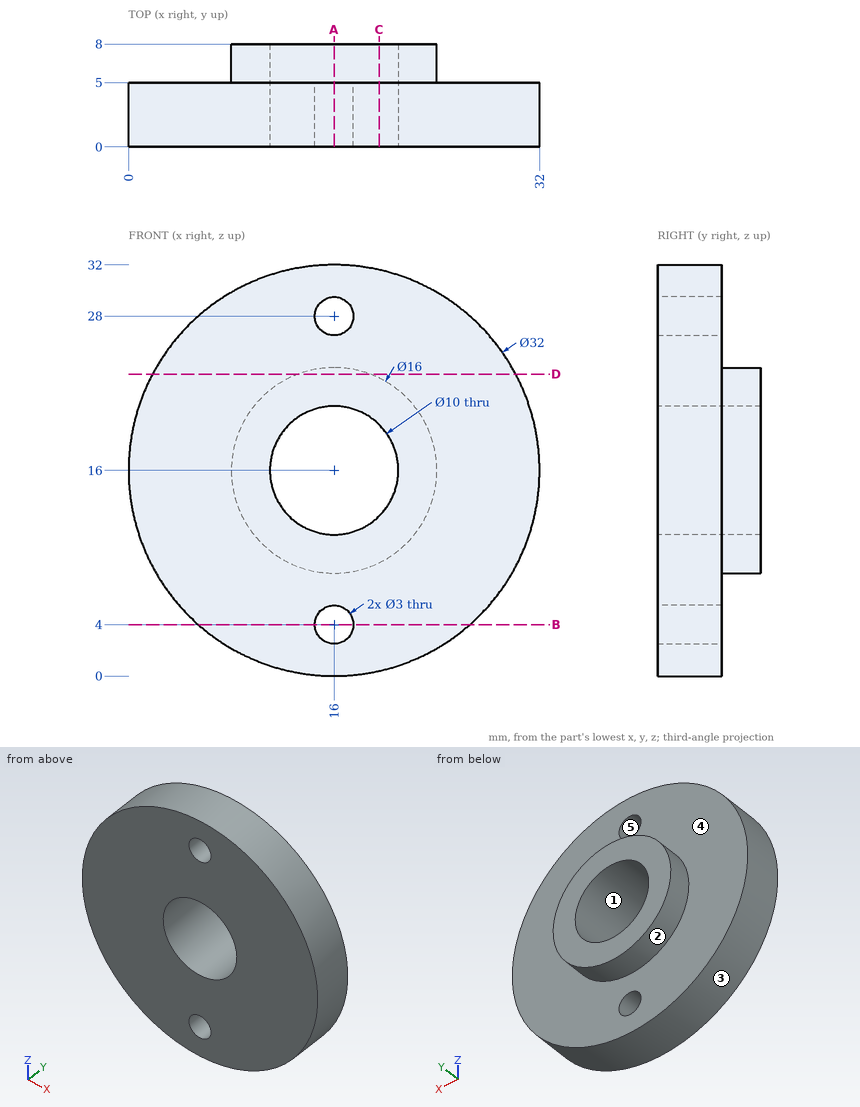
Can you work these out from the drawing? Everything is in mm from the part's minimum corner. A direction names the side the tool comes from. Round coordinates to 2 decimals unless told otherwise and drop trailing zeros. Write each loop counter-clockwise with the first axis right and the second up, starting at its lowest first coordinate (ties: lowest second). Pieces come first, ordered by that corner, then holes. Notation, with made-up numbers: (-8.75, 19.5) - (29.25, 19.5) arc R14 cw to (29.25, 35.5) - close; hole circle Ø9 at (-36.75, 26). An arc over 180 degrees is marked (long way). Write each question's results on one line, items separated by ' | '. Start each with the question number.
1) Which directions (+Z, -Z, +X, -X, +Y, -Y) give clear straight access to the entire face, cutting with the end or side of a thin tool? Please do the marked faces 1 and 2.
2) Please list where these lines run through material, in increasing order: line 1 (Y direction, x = 19, z = 27); line 2 (X direction, y = 3.75, z = 16); line 3 (X direction, y = 1.9, z = 28).
3) We'd pull the mould along Z, two halves only. Please class the marked faces 3, 4 and 5: released by +Z, released by -Z, zero draft, split by the parting line, or undercut.
4) Suppose I cut it at A-A (x = 16). List the corners of the cut face in (y, z) for me, and give its area (3 significant figures).
5) Suppose I cut it at B-B (z = 4). List the corners of the cut face in (x, y) for me.
6) For pin 1 Ø3 at (y, z) = (5, 4.5) entering from +X; pin 2 Ø3 at (x, y) = (12, 1.5) entering from +Z; pin 3 Ø4 at (x, y) = (26, 2) entering from +Z, each with a flat end and sliding along its axis, tell me the tip position at first contact or that it passes through.
7) Suppose I cut it at D-D (z = 23.5). List the corners of the cut face in (x, y) for me.
8) Suppose I cut it at C-C (x = 19.5). List the corners of the cut face in (y, z) for me.
Here are the results:
1) face 1: +Y, -Y | face 2: +Y
2) line 1: y = 0 to 5 | line 2: x = 0 to 11, 21 to 32 | line 3: x = 5.42 to 14.5, 17.5 to 26.58
3) face 3: split by the parting line | face 4: zero draft | face 5: undercut
4) outline: (0, 0) - (5, 0) - (5, 2.5) - (0, 2.5) - close; (0, 5.5) - (5, 5.5) - (5, 8) - (8, 8) - (8, 11) - (0, 11) - close; (0, 21) - (8, 21) - (8, 24) - (5, 24) - (5, 26.5) - (0, 26.5) - close; (0, 29.5) - (5, 29.5) - (5, 32) - (0, 32) - close | area: 98.0 mm2
5) outline: (5.42, 0) - (14.5, 0) - (14.5, 5) - (5.42, 5) - close; (17.5, 0) - (26.58, 0) - (26.58, 5) - (17.5, 5) - close
6) pin 1: stops at x = 28.49 | pin 2: stops at z = 31.8 | pin 3: stops at z = 29.86
7) outline: (1.87, 0) - (30.13, 0) - (30.13, 5) - (18.78, 5) - (18.78, 8) - (13.22, 8) - (13.22, 5) - (1.87, 5) - close
8) outline: (0, 0.39) - (5, 0.39) - (5, 8.81) - (8, 8.81) - (8, 12.43) - (0, 12.43) - close; (0, 19.57) - (8, 19.57) - (8, 23.19) - (5, 23.19) - (5, 31.61) - (0, 31.61) - close
